Verification items for this drawing (mm, ordinates from the low corner). Coordinates: 2 decimals unless noted, no trailing zeros. Order: outer loops, then holes, each group sorted by start corner. A loop starts at its lowest first (then second) coordinate and runs counter-clockwise, first axis right, second up. Notation, with made-up numbers: M -6,10.5 L 19,10.5 A32 cw 19,37.5 Z; hole C 77,-20.75 d4. An arc over 180 degrees is marked long. Write item = value, one per line.
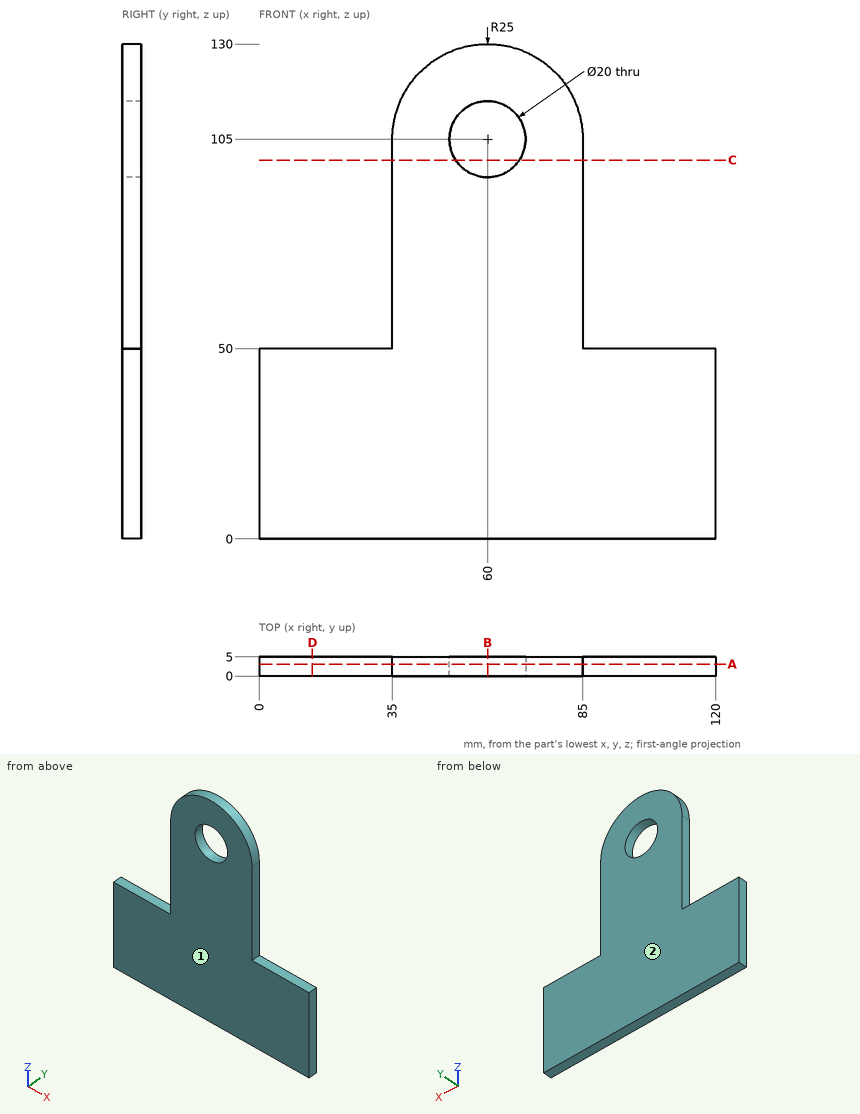
Item 1: Release check for a two-part mould opening along Y. For the marked faces 1 and 2 record: pulls with the +Y half, pulls with the -Y half, needs draft (parallel to the pull), parting line crosses it, or undercut.
Report:
face_1 = pulls with the -Y half
face_2 = pulls with the +Y half
Item 2: Sectioned sample at B-B, the plane x = 60. Enter the section's corners in (y, z).
Report:
outline = M 0,0 L 5,0 L 5,95 L 0,95 Z; M 0,115 L 5,115 L 5,130 L 0,130 Z
Item 3: Sectioned sample at C-C, the plane z = 99.5. Enter the section's corners in (x, y), then the cut area to 3 significant figures.
Report:
outline = M 35,0 L 51.65,0 L 51.65,5 L 35,5 Z; M 68.35,0 L 85,0 L 85,5 L 68.35,5 Z
area = 166 mm^2
Item 4: Scan lines: L1, parallel to X at y = 3.5, z = 105; L2, parallel to Z at x = 60, y = 2.85; L3, parallel to Z at x = 91.5, y = 2.8. Record each from-to range of solid material in increasing order. Write a range as from..to.
Report:
L1 = 35..50, 70..85
L2 = 0..95, 115..130
L3 = 0..50
Item 5: Gauge pin test, flat ends, axial feed: pin 1 (2 mm diameter, centred on x = 14.5, y = 3, fed in from -Z); pin 2 (2 mm diameter, centred on x = 33, y = 4, fed in from +Z); pin 3 (1.5 mm diameter, centred on y = 1.5, z = 74.5, fed in from +X); pin 4 (8 mm diameter, centred on x = 30, z = 96, fed in from -Y). Record the tip position at first contact, or that the pin passes through.
Report:
pin_1 = 0
pin_2 = 50
pin_3 = 85
pin_4 = through
Item 6: Sectioned sample at D-D, the plane x = 14. Enter the section's corners in (y, z).
Report:
outline = M 0,0 L 5,0 L 5,50 L 0,50 Z
Item 7: Sectioned sample at A-A, the plane y = 3.1. Enter the section's corners in (x, z), then the cut area to 3 significant figures.
Report:
outline = M 0,0 L 120,0 L 120,50 L 85,50 L 85,105 A25 ccw 35,105 L 35,50 L 0,50 Z; hole C 60,105 d20
area = 9,420 mm^2
